Source: CAD feature listing. Evaluate the final solid. Frame: model axes, mm. Face numbers are marked on the shaded views. A direction names the side the tool comes from. Give positions to 0.01 mm unless a question says otherwise; leave off trailing zeros. Order: outer loops, then holes, each group sorted by start corner. A loop starts at its lowest first (then second) coordinate and runs counter-clockwise, first axis right, second up. Notation, with made-up numbers: (51, -4.5) -> (78, -4.5) arc R25 cw to (78, 20.5) -> close; hole circle Ø11 at (48, 32.25). An arc over 180 degrees is marked (long way). Use one line per item in the form item = value. Start each with the question number.
from build123d import *

# Parameters (mm, degrees)
SKETCH1_W           = 68.58
SKETCH1_H           = 50.8
BOSS_EXTRUDE1_DEPTH = 19.05
SKETCH2_W           = 45.72
SKETCH2_H           = 21.59
CUT_EXTRUDE1_DEPTH  = 16.51


with BuildPart() as part:
    # Sketch1 → Boss-Extrude1 (new body)
    with BuildSketch(Plane.YZ):
        with Locations((34.29, 25.4)):
            Rectangle(SKETCH1_W, SKETCH1_H)
    extrude(amount=BOSS_EXTRUDE1_DEPTH)

    # Sketch2 → Cut-Extrude1 (cut)
    with BuildSketch(Plane.YZ.offset(19.05)):
        with Locations((34.29, 40.005)):
            Rectangle(SKETCH2_W, SKETCH2_H)
    extrude(amount=-CUT_EXTRUDE1_DEPTH, mode=Mode.SUBTRACT)


solid = part.part
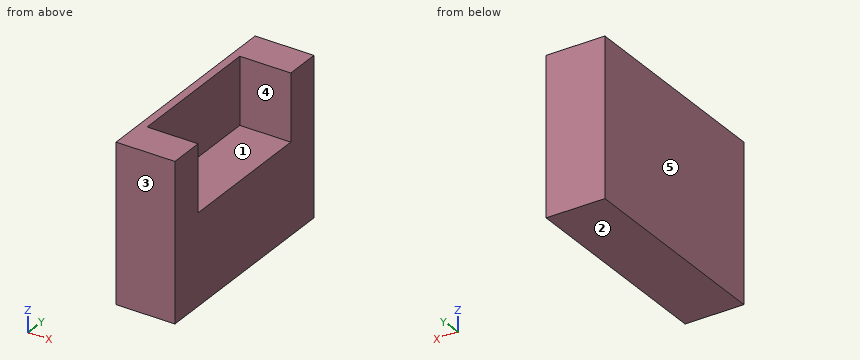
1) Reachability of the marked faces 1 and 2 from +Z, -Z, +X, -X, +Y, -Y: full face, straight path, thin tool, end or side. Return the list, or none.
2) Pin query (flat end, axial travel): pin 1 (17.5 mm diameter, centred on y = 27.5, z = 42, fed in from +X); pin 2 (6 mm diameter, centred on y = 47.5, z = 5.5, fed in from -X); pin 3 (10 mm diameter, centred on x = 13.5, y = 40.5, fed in from +Z). Return the tip coordinate at first contact, or that it passes through.
3) Cut plane C-C, the plane y = 18. Return the cut outline in (x, z).
4) Cut plane B-B, the plane z = 44. Return the cut outline in (x, y).
5) Draft query along Y for the marked faces 3, 4 and 5. Return one class per face: +Y half, -Y half, draft (parallel to the pull), parting line (faces both ways), or undercut.
6) Material intervals for probe 1 along Y at (x, z) = (14, 41); probe 2 along Z at (x, y) = (15.75, 19.5); probe 3 along X at (y, z) = (33.5, 30.5), sorted ascending.
7) Cut plane A-A, the plane x = 17.5. Return the cut outline in (y, z).
Output values:
q1.face_1 = +Z, +X
q1.face_2 = -Z, +X, -X, +Y, -Y
q2.pin_1 = 2.54
q2.pin_2 = 0
q2.pin_3 = 29.21
q3.outline = (0, 0) -> (19.05, 0) -> (19.05, 29.21) -> (2.54, 29.21) -> (2.54, 50.8) -> (0, 50.8) -> close
q4.outline = (0, 0) -> (19.05, 0) -> (19.05, 11.43) -> (2.54, 11.43) -> (2.54, 57.15) -> (19.05, 57.15) -> (19.05, 68.58) -> (0, 68.58) -> close
q5.face_3 = -Y half
q5.face_4 = undercut
q5.face_5 = draft
q6.probe_1 = 0 to 11.43, 57.15 to 68.58
q6.probe_2 = 0 to 29.21
q6.probe_3 = 0 to 2.54
q7.outline = (0, 0) -> (68.58, 0) -> (68.58, 50.8) -> (57.15, 50.8) -> (57.15, 29.21) -> (11.43, 29.21) -> (11.43, 50.8) -> (0, 50.8) -> close
